CAD build for the part. Positions are in the model's coordinates, mm. A direction names the side the tool comes from. Round coordinates to 2 decimals unless told otherwise and drop trailing zeros. Loops run counter-clockwise (first coordinate to the right, second up) from the corner with the lowest first, then second, coordinate; pieces in that order, holes last. Notation, with made-up numbers: M 19.5,-37 L 31.5,-37 A31 cw 31.5,-8 Z; hole C 72,77.25 d1. An arc over 180 degrees is marked long. Use a Markdown table: item, result. Add a question column.
(1) Wall check: L1, parallel to X at y = -22.5, z = 4; L2, parallel to Y at x = 5, z = 10; L3, parallel to Y at x = -7.5, z = 15.5. Give the ranges that are in metal, low to high.
(2) Band-saw the part on A-A, the plane x = 7.5. Write the cut outline in (y, z) (1 decimal).
(3) Two-plate mould, pull along Z, no slides. Class faces 4 (the face through (-0.34, 50.27, 20.29)), 5 (the face through (0.336, -70.536, 7.757)), 6 (the face through (26.5, 0, 13)): released by +Z, released by -Z, zero draft, split by the parting line, or undercut.
(4) Flat gauge pins, fed straight in: P1, Ø16.5, axis at x = 4, z = 6.5, coming from the -Y side; P2, Ø2, axis at x = 10.5, z = 14, coming from the -Y side; P3, Ø1.5, axis at x = 4, y = 38.5, coming from the -Z side. Where does each tip first touch, or does it go through?
(5) Which spindle directions (+Z, -Z, +X, -X, +Y, -Y) get a long thin tool onto all of the face, cutting with end or side? Do faces 1 (the face through (-0.34, -67.91, 17.41)), 2 (the face through (25.787, 70.956, 7.657)), 3 (the face through (27.574, 72.704, 7.657)). Say none if no direction does.
from build123d import *

# Parameters (mm, degrees)
F1_DEPTH = 29
F2_F1_R  = 5
F2_F2_R  = 5
F3_T     = -2.5


with BuildPart() as f1:
    # F0 (on Right) → F1 (new body, symmetric)
    with BuildSketch(Plane.YZ):
        with BuildLine():
            ThreePointArc((-71.5784906799, 19.7169460854), (-70.4874573475, 9.8584730427), (-71.5784906799, 0))
            Line((-71.5784906799, 0), (-54.9704477794, 0))
            ThreePointArc((-54.9704477794, 0), (-43.1382882132, 14), (-31.306128647, 0))
            Line((-31.306128647, 0), (16.2495522206, 0))
            ThreePointArc((16.2495522206, 0), (28.0817117868, 14), (39.913871353, 0))
            Line((39.913871353, 0), (74.2074146826, 0))
            Line((74.2074146826, 0), (74.2074146826, 19.4779538288))
            Line((74.2074146826, 19.4779538288), (51.0250648113, 22.5848669347))
            ThreePointArc((51.0250648113, 22.5848669347), (-2.8965217341, 36.6382547678), (-56.9998987666, 23.3018459996))
            Line((-56.9998987666, 23.3018459996), (-71.5784906799, 19.7169460854))
        make_face()
        with BuildLine():
            ThreePointArc((-31.306128647, 0), (-43.1382882132, 14), (-54.9704477794, 0))
            Line((-54.9704477794, 0), (-31.306128647, 0))
        make_face()
        with BuildLine():
            ThreePointArc((39.913871353, 0), (28.0817117868, 14), (16.2495522206, 0))
            Line((16.2495522206, 0), (39.913871353, 0))
        make_face()
    extrude(amount=F1_DEPTH, both=True)

    # F2: fillet of radius 5 on 10 edges, made by hand

    # F2_f1
    f2_f1_edges = [f1.edges().sort_by_distance(p)[0] for p in [
        (0, -56.9998987666, 23.3018459996),
        (0, 51.0250648113, 22.5848669347),
    ]]
    fillet(f2_f1_edges, radius=F2_F1_R)

    # F2_f2
    f2_f2_edges = [f1.edges().sort_by_distance(p)[0] for p in [
        (0, -71.5784906799, 19.7169460854),
        (-29, -70.4874573475, 9.8584730427),
        (29, -70.4874573475, 9.8584730427),
        (-29, -3.0466412139, 36.6391517316),
        (29, -3.0466412139, 36.6391517316),
        (0, 74.2074146826, 19.4779538288),
        (29, 74.2074146826, 9.7389769144),
        (-29, 74.2074146826, 9.7389769144),
        (29, 51.0608622621, 22.6625045572),
        (29, -57.0196487491, 23.3351165373),
        (-29, 51.0608622621, 22.6625045572),
        (-29, -57.0196487491, 23.3351165373),
    ]]
    fillet(f2_f2_edges, radius=F2_F2_R)

    # F3
    f3_openings = [f1.faces().sort_by_distance(p)[0] for p in [
        (0, 1.316584, 0),
    ]]
    offset(amount=F3_T, openings=f3_openings, kind=Kind.INTERSECTION)


solid = f1.part
Return value:
| question | item | result |
|---|---|---|
| 1 | L1 | -29 to -26.5, 26.5 to 29 |
| 1 | L2 | -70.49 to -67.99, 71.71 to 74.21 |
| 1 | L3 | -70.84 to -68.32, 71.68 to 74.19 |
| 2 | outline | M -71.6,0 L -69,0 A47.6 ccw -68.3,15.7 A2.5 cw -66.5,18.4 L -57,20.7 A7.5 ccw -55.3,21.4 A110.9 cw 49,20.8 A7.5 ccw 51.6,20 L 69.5,17.6 A2.5 cw 71.7,15.1 L 71.7,0 L 74.2,0 L 74.2,15.1 A5 ccw 69.9,20.1 L 51.9,22.5 A5 cw 50.2,23 A113.4 ccw -56.5,23.6 A5 cw -57.6,23.2 L -67.1,20.8 A5 ccw -70.8,15.4 A45.1 cw Z |
| 3 | face 4 | released by -Z |
| 3 | face 5 | undercut |
| 3 | face 6 | zero draft |
| 4 | P1 | y = -71.58 |
| 4 | P2 | y = -70.78 |
| 4 | P3 | z = 25.5 |
| 5 | face 1 | none |
| 5 | face 2 | -Z |
| 5 | face 3 | +Z, -Z, +X, +Y |
